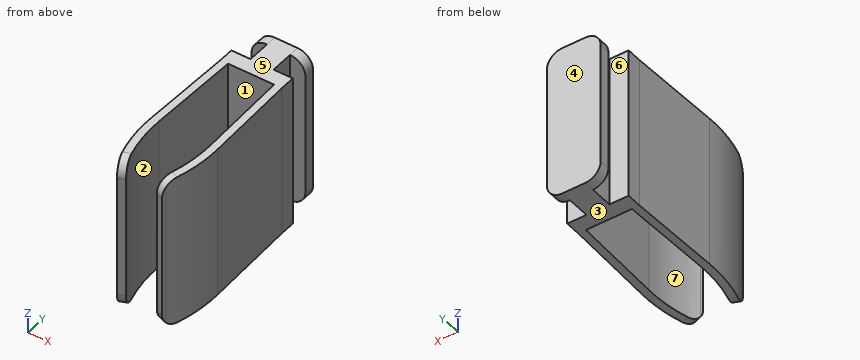
```python
from build123d import *

# Parameters (mm, degrees)
F0_W     = 7
F0_H     = 20
F1_DEPTH = 1.4
F2_W     = 3
F2_H     = 20
F3_DEPTH = 3
F4_W     = 8
F4_H     = 20
F5_DEPTH = 2
F8_DEPTH = 20
F9_R     = 20
F10_R    = 2


# Not quite as in the source:
# - a feature of the source that left no trace in its solid (it failed there, or was rolled back) is left out


with BuildPart() as f1:
    # F0 (on Front) → F1 (new body)
    with BuildSketch(Plane.XZ):
        Rectangle(F0_W, F0_H)
    extrude(amount=F1_DEPTH)

    # F2 (on face) → F3 (join)
    with BuildSketch(Plane.XZ.offset(1.4)):
        Rectangle(F2_W, F2_H)
    extrude(amount=F3_DEPTH)

    # F4 (on face) → F5 (join)
    with BuildSketch(Plane.XZ.offset(4.4)):
        Rectangle(F4_W, F4_H)
    extrude(amount=F5_DEPTH)

    # F7 (on face) → F8 (join, through all)
    with BuildSketch(Plane.XY.offset(10)):
        Polygon((-2.9995108826, -6.4), (-4, -6.4), (-4.5057272064, -22.5674550383), (-2.9367871525, -26.7512951822), (-2, -26.4), (-3.5, -22.4), align=None)
        Polygon((4, -6.4), (2.9995108826, -6.4), (3.5, -22.4), (2, -26.4), (2.9367871525, -26.7512951822), (4.5057272064, -22.5674550383), align=None)
    extrude(amount=-F8_DEPTH)

    # F9
    f9_edges = [f1.edges().sort_by_distance(p)[0] for p in [
        (-3.5, -22.4, 0),
        (3.5, -22.4, 0),
        (4.505727, -22.567455, 0),
        (-4.505727, -22.567455, 0),
    ]]
    fillet(f9_edges, radius=F9_R)

    # F10
    f10_edges = [f1.edges().sort_by_distance(p)[0] for p in [
        (-2.468394, -26.575648, 10),
        (2.468394, -26.575648, 10),
        (-2.468394, -26.575648, -10),
        (2.468394, -26.575648, -10),
        (-3.5, -0.7, -10),
        (3.5, -0.7, -10),
        (-3.5, -0.7, 10),
        (3.5, -0.7, 10),
    ]]
    fillet(f10_edges, radius=F10_R)


solid = f1.part
```
The listing builds one solid part. Answer for the finished solid, in the listing's coordinates (mm). Face numbers are marked on the shaded views. A direction names the side the tool comes from. Give positions to 0.01 mm unless a question says otherwise; leave off trailing zeros. Order: outer loops, then holes, each group sorted by start corner. A loop starts at its lowest first (then second) coordinate and runs counter-clockwise, first axis right, second up. Notation, with made-up numbers: M 70,17 L 82,17 A18 ccw 82,32 Z; hole C 24.25,46.25 d4. An arc over 180 degrees is marked long. Put each result on its own line as item: value. Start each with the question number.
Item 1: The part is cut by section B-B, the plane z = -0.75. Determine the outline of the cut face in (x, y).
Item 2: The part is cut by section D-D, the plane y = -1.75. Determine the outline of the cut face in (x, z), and give its area (3 significant figures).
Item 3: For a pull along Y with two mould halves and no side action, classify the marked faces 1, 2, 3 and 4 as +Y half, -Y half, draft (parallel to the pull), parting line (faces both ways), or undercut.
Item 4: Find the intervals of material crossed by line 1 along Y through (x, z) = (1.75, -0.5); line 2 along Y through (x, z) = (0, 8); line 3 along X through (y, z) = (-4.75, -3), in increasing order.
Item 5: The part is cut by section C-C, the plane x = 0. Determine the outline of the cut face in (y, z), and give its area (3 significant figures).
Item 6: Flat-ended cylindrical pins translate along their axes: P1, Ø2, axis at y = -21, z = 0.5, coming from the -X side; P2, Ø1.5, axis at y = -2.5, z = 0, coming from the +X side; P3, Ø0.7, axis at y = -1, z = 1.5, coming from the +X side; P4, Ø2, axis at x = -3.5, y = -3, coming from the +Z side. Find the tip coordinate at first contact, or state that the pin passes through.
Item 7: Which of the six approach directions +Z, -Z, +X, -X, +Y, -Y give full straight-line access (tool end or side, diameter ignored) to the marked faces 5, 6 and 7?
Item 8: The part is cut by section A-A, the plane y = -20.5. Determine the outline of the cut face in (x, z), and give its area (3 significant figures).
Answer key:
1. outline: M -4.38,-18.62 A20 ccw -3.12,-26.27 L -2.94,-26.75 L -2,-26.4 L -2.11,-26.1 A20 cw -3.38,-18.45 L -3,-6.4 L 3,-6.4 L 3.38,-18.45 A20 cw 2.11,-26.1 L 2,-26.4 L 2.94,-26.75 L 3.12,-26.27 A20 ccw 4.38,-18.62 L 4,-6.4 L 4,-4.4 L 1.5,-4.4 L 1.5,-1.4 L 3.5,-1.4 L 3.5,0 L -3.5,0 L -3.5,-1.4 L -1.5,-1.4 L -1.5,-4.4 L -4,-4.4 L -4,-6.4 Z
2. outline: M -1.5,-10 L 1.5,-10 L 1.5,10 L -1.5,10 Z
2. area: 60.0 mm²
3. face 1: undercut
3. face 2: undercut
3. face 3: draft
3. face 4: +Y half
4. line 1: y = -6.4 to -4.4, -1.4 to 0
4. line 2: y = -6.4 to 0
4. line 3: x = -4 to 4
5. outline: M -6.4,-10 L 0,-10 L 0,10 L -6.4,10 Z
5. area: 128 mm²
6. P1: stops at x = -4.38
6. P2: stops at x = 1.5
6. P3: stops at x = 3.5
6. P4: passes through
7. face 5: +Z, +X, -X, +Y, -Y
7. face 6: +Z, -Z, -X
7. face 7: +Z, -Z
8. outline: M -4.35,-10 L -3.34,-10 L -3.34,10 L -4.35,10 Z; M 3.34,-10 L 4.35,-10 L 4.35,10 L 3.34,10 Z
8. area: 40.7 mm²
